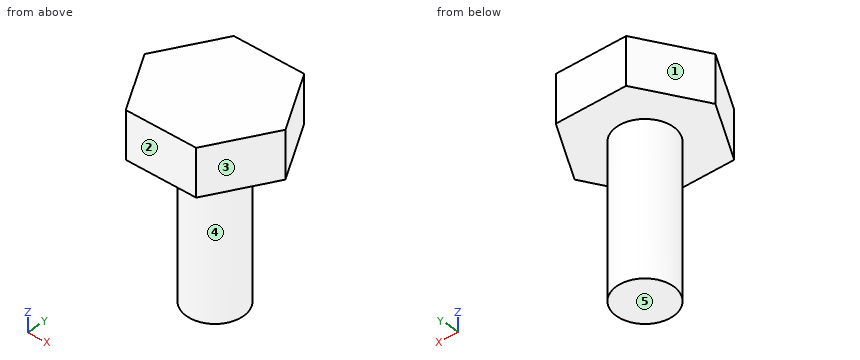
```python
from build123d import *

# Parameters (mm, degrees)
BOSS_EXTRUDE1_DEPTH = 6.35
SKETCH2_R           = 3.81
BOSS_EXTRUDE2_DEPTH = 20.32


with BuildPart() as part:
    # Sketch1 → Boss-Extrude1 (new body)
    with BuildSketch(Plane.XY):
        Polygon((4.766026472, -8.255), (9.532052944, 0), (4.766026472, 8.255), (-4.766026472, 8.255), (-9.532052944, 0), (-4.766026472, -8.255), align=None)
    extrude(amount=BOSS_EXTRUDE1_DEPTH)

    # Sketch2 → Boss-Extrude2 (add)
    with BuildSketch(Plane(origin=(0, 0, 0), x_dir=(-1, 0, 0), z_dir=(0, 0, -1))):
        with Locations(Location((0, 0, 0), (0, 0, 180))):
            Circle(SKETCH2_R)
    extrude(amount=BOSS_EXTRUDE2_DEPTH)


solid = part.part
```
The model under review builds one solid part; all positions refer to its coordinate system, in mm. Face numbers are marked on the shaded views. A direction names the side the tool comes from. Round coordinates to 2 decimals unless told otherwise and drop trailing zeros. Order: outer loops, then holes, each group sorted by start corner. A loop starts at its lowest first (then second) coordinate and runs counter-clockwise, first axis right, second up.
Item 1: Add section B-B, the plane x = 0. State the section outline as (y, z) points (3 decimals).
Working result:
outline: (-8.255, 0) - (-3.81, 0) - (-3.81, -20.32) - (3.81, -20.32) - (3.81, 0) - (8.255, 0) - (8.255, 6.35) - (-8.255, 6.35) - close
Item 2: Add section C-C, the plane y = -2. State the section outline as (x, z) points.
Working result:
outline: (-8.38, 0) - (-3.24, 0) - (-3.24, -20.32) - (3.24, -20.32) - (3.24, 0) - (8.38, 0) - (8.38, 6.35) - (-8.38, 6.35) - close
Item 3: Draft analysis for pull direction X (two halves, no side actions). For the marked faces 1, 2 and 3, state which applies: released by +X, released by -X, zero draft, split by the parting line, or undercut.
Working result:
face 1: released by -X
face 2: zero draft
face 3: released by +X
Item 4: Machinability: for the marked faces 4 and 5, which of the approach directions +Z, -Z, +X, -X, +Y, -Y give a long, thin tool a straight path to every point of the face, cutting with its end or side? Answer none if there is none.
Working result:
face 4: -Z
face 5: -Z, +X, -X, +Y, -Y
Item 5: Add section A-A, the plane z = 4. State the section outline as (x, y) points (3 decimals), and give its area (3 significant figures).
Working result:
outline: (-9.532, 0) - (-4.766, -8.255) - (4.766, -8.255) - (9.532, 0) - (4.766, 8.255) - (-4.766, 8.255) - close
area: 236 mm2
Item 6: To check wall thickness, follow probe 1 along Z at (x, y) = (-2.75, -6); probe 2 along Y at (x, z) = (1.5, -9.25); probe 3 along X at (y, z) = (-1.25, -7.75). State the ranges of each line that lie inside material, in increasing order.
Working result:
probe 1: z = 0 to 6.35
probe 2: y = -3.5 to 3.5
probe 3: x = -3.6 to 3.6
Item 7: For pin 1 (3 mm diameter, centred on x = 6.5, z = 2.5, fed in from -Y); pin 2 (3 mm diameter, centred on y = 0.5, z = 0.5, fed in from +X); pin 3 (4 mm diameter, centred on y = -5.5, z = -4, fed in from -X); pin 4 (4 mm diameter, centred on x = 7, z = -10, fed in from +Y), all flat-tipped, find the tip position at first contact; note any pin that passes through.
Working result:
pin 1: stops at y = -7.85
pin 2: stops at x = 9.53
pin 3: stops at x = -1.51
pin 4: passes through
Item 8: Add section D-D, the plane z = -14. State the section outline as (x, y) points.
Working result:
outline: circle Ø7.62 at (0, 0)
